Can you work these out from the model? Positions are in its coordinate system, mm. A direction names the side the tool comes from. Give positions to 0.01 mm unless a question says otherwise; leave off trailing zeros.
```python
from build123d import *

# Parameters (mm, degrees)
F1_DEPTH = 25
F2_W     = 28.6602540378
F2_H     = 25
F3_DEPTH = 200
F3_TAPER = -3


with BuildPart() as f1:
    # F0 (on Top) → F1 (new body)
    with BuildSketch(Plane.XY):
        Polygon((0, 10), (0, 0), (28.6602540378, 0), (28.6602540378, 39.6410161514), (8.6602540378, 5), align=None)
    extrude(amount=F1_DEPTH)

    # F2 (on face) → F3 (join)
    with BuildSketch(Plane.XZ):
        with Locations((14.3301270189, 12.5)):
            Rectangle(F2_W, F2_H)
    extrude(amount=F3_DEPTH, taper=F3_TAPER)


solid = f1.part
```
1) If I drill on line 1 (Z direction, x = 17, y = -144); line 2 (Y direction, x = 3, z = 15); line 3 (Z direction, x = 24, y = -134), over which ranges is the centre line in solid material (lowest first)?
2) We'd pull the mould along X, two halves only. Please class faces 1 (the face through (0, 5, 12)), 2 (the face through (28.66, 20, 12)), 3 (the face through (14, -200, 13)), 4 (the face through (4.391, 7.465, 12.325)): +X half, -X half, draft (parallel to the pull), parting line (faces both ways), or undercut.
3) Which directions (+Z, -Z, +X, -X, +Y, -Y) give clear straight access to the entire face, cutting with the end or side of a thin tool? Please do faces 5 (the face through (17, 11, 0)), 6 (the face through (17, 11, 25)).
4) I'm going to push flat-ended pins straight in: pin 1 Ø14.5 at (x, y) = (17, 20.5) entering from -Z; pin 2 Ø8 at (y, z) = (-134, 8.5) entering from +X; pin 3 Ø1 at (y, z) = (-36, 7.5) entering from +X. Where does each tip first touch, or does it pass through?
Results:
1. line 1: z = -7.55 to 32.55
1. line 2: y = -200 to 8.27
1. line 3: z = -7.02 to 32.02
2. face 1: -X half
2. face 2: +X half
2. face 3: draft
2. face 4: undercut
3. face 5: -Z, +X, -X, +Y
3. face 6: +Z, +X, -X, +Y
4. pin 1: stops at z = 0
4. pin 2: stops at x = 35.89
4. pin 3: stops at x = 30.57
